Source: CAD feature listing. Evaluate the final solid. Frame: model axes, mm. A direction names the side the tool comes from. Coordinates: 2 decimals unless noted, no trailing zeros. Order: outer loops, then holes, each group sorted by start corner. A loop starts at its lowest first (then second) coordinate and runs counter-clockwise, first axis right, second up.
Item 1: Reachability of faces 4 (the cylindrical face through (-6.4, 0.1, -3.5)), 5 (the cylindrical face through (0, 2, -15)), 6 (the cylindrical face through (6.4, 0.1, -3.5)), 7 (the cylindrical face through (0.1, -6.4, -3.5)) from +Z, -Z, +X, -X, +Y, -Y: full face, straight path, thin tool, end or side. Return the list, or none.
Item 2: Section D-D on z = -8.75. Return the cut outline in (x, y).
Item 3: Section A-A on x = 0. Return the cut outline in (y, z).
Item 4: Ray query, line 1 (Z direction, x = -3.25, y = -7.5); line 2 (Z direction, x = -3, y = -5); line 3 (X direction, y = -2, z = -8.75). Return the intervals inside material, ascending.
Item 5: Contact query for flat-ended pins moving along their axis: P1, Ø0.6, axis at x = -9, y = 9, coming from the -Z side; P2, Ø10, axis at y = -2, z = -12.5, coming from the +X side; P3, Ø4, axis at x = -6.5, z = -10, coming from the +Y side; P4, Ø10, axis at x = -1.5, z = -4.5, coming from the +Y side. Output: stop coordinate, or through.
Item 6: Mould query, pull axis X, two halves, no side actions, for faces 1 (the cylindrical face through (0.1, 6.5, -3.5)), 2 (the flat face through (0, 0, -18)), 3 (the flat face through (-9.25, 0, 1)). Classes: released by +X, released by -X, zero draft, split by the parting line, or undercut.
Item 7: Section C-C on z = -15.25. Return the cut outline in (x, y).
from build123d import *

# Parameters (mm, degrees)
F0_W          = 18.5
F0_H          = 11
F1_DEPTH      = 9.25
F2_DEPTH      = 9.25
F3_R          = 19
F5_DEPTH      = 25.4
F6_DEPTH      = 25.4
F4_R          = 19
F7_DEPTH      = 25.4
F8_DEPTH      = 25.4
F9_R          = 4
F10_DEPTH     = 3.45753
F11_DEPTH     = 7.5
F12_T1_DEPTH  = 11.75
F12_T3_DEPTH  = 17.5
F12_T5_DEPTH  = 17.5
F12_S9_W      = 0.5
F12_S9_H      = 0.5
F12_T10_DEPTH = 0.5
F12_S15_W     = 0.5
F12_S15_H     = 0.5
F12_T16_DEPTH = 0.5
F12_S21_W     = 0.5
F12_S21_H     = 0.5
F12_T22_DEPTH = 0.5
F12_S27_W     = 0.5
F12_S27_H     = 0.5
F12_T28_DEPTH = 0.5
F12_T34_ANGLE = 60.5906744424
F12_T36_ANGLE = 60.5906744424
F12_T38_ANGLE = 60.5906744424
F12_T40_ANGLE = 60.5906744424
F13_R         = 1.9993297739
F14_DEPTH     = 5


# Not quite as in the source:
# - a fillet or chamfer that OpenCascade refuses, or shapes differently, is made with other operations: its cross-section is extruded or revolved along the edge and cut away or added
# - a feature names something its author has since deleted; it is built from what else it names


with BuildPart() as f1:
    # F0 (on Front) → F1 (new body)
    with BuildSketch(Plane.XZ):
        Rectangle(F0_W, F0_H)
    extrude(amount=-F1_DEPTH)

    # F0 (on Front) → F2 (join)
    with BuildSketch(Plane.XZ):
        Rectangle(F0_W, F0_H)
    extrude(amount=F2_DEPTH)

    # F3 (on Front) → F5 (cut)
    with BuildSketch(Plane.XZ):
        with Locations((0, -22.5)):
            Circle(F3_R)
    extrude(amount=-F5_DEPTH, mode=Mode.SUBTRACT)

    # F3 (on Front) → F6 (cut)
    with BuildSketch(Plane.XZ):
        with Locations((0, -22.5)):
            Circle(F3_R)
    extrude(amount=F6_DEPTH, mode=Mode.SUBTRACT)

    # F4 (on Right) → F7 (cut)
    with BuildSketch(Plane.YZ):
        with Locations((0, -22.5)):
            Circle(F4_R)
    extrude(amount=-F7_DEPTH, mode=Mode.SUBTRACT)

    # F4 (on Right) → F8 (cut)
    with BuildSketch(Plane.YZ):
        with Locations((0, -22.5)):
            Circle(F4_R)
    extrude(amount=F8_DEPTH, mode=Mode.SUBTRACT)

    # F9 (on face) → F10 (join)
    with BuildSketch(Plane(origin=(0, 0, -5.5), x_dir=(1, 0, 0), z_dir=(0, 0, -1))):
        Circle(F9_R)
    extrude(amount=-F10_DEPTH)

    # F11 (add): a face of the model
    f11_faces = [f1.faces().sort_by_distance(p)[0] for p in [
        (0, 0, -5.5),
    ]]
    extrude(f11_faces, amount=F11_DEPTH)

    # F12: fillet of radius 0.5 on 13 edges, made by hand

    # F12_s2 → F12_t1 (cut)
    with BuildSketch(Plane.XY.offset(-6.75)):
        with BuildLine():
            ThreePointArc((9.25, -8.75), (9.1035533906, -9.1035533906), (8.75, -9.25))
            Line((8.75, -9.25), (9.25, -9.25))
            Line((9.25, -9.25), (9.25, -8.75))
        make_face()
        with BuildLine():
            ThreePointArc((-9.25, -8.75), (-9.1035533906, -9.1035533906), (-8.75, -9.25))
            Line((-8.75, -9.25), (-9.25, -9.25))
            Line((-9.25, -9.25), (-9.25, -8.75))
        make_face()
        with BuildLine():
            ThreePointArc((9.25, 8.75), (9.1035533906, 9.1035533906), (8.75, 9.25))
            Line((8.75, 9.25), (9.25, 9.25))
            Line((9.25, 9.25), (9.25, 8.75))
        make_face()
        with BuildLine():
            ThreePointArc((-8.75, 9.25), (-9.1035533906, 9.1035533906), (-9.25, 8.75))
            Line((-9.25, 8.75), (-9.25, 9.25))
            Line((-9.25, 9.25), (-8.75, 9.25))
        make_face()
    extrude(amount=F12_T1_DEPTH, mode=Mode.SUBTRACT)

    # F12_s4 → F12_t3 (cut)
    with BuildSketch(Plane.YZ.offset(-8.75)):
        with BuildLine():
            ThreePointArc((-8.75, 5.5), (-9.1035533906, 5.3535533906), (-9.25, 5))
            Line((-9.25, 5), (-9.25, 5.5))
            Line((-9.25, 5.5), (-8.75, 5.5))
        make_face()
        with BuildLine():
            ThreePointArc((9.25, 5), (9.1035533906, 5.3535533906), (8.75, 5.5))
            Line((8.75, 5.5), (9.25, 5.5))
            Line((9.25, 5.5), (9.25, 5))
        make_face()
    extrude(amount=F12_T3_DEPTH, mode=Mode.SUBTRACT)

    # F12_s6 → F12_t5 (cut)
    with BuildSketch(Plane.XZ.offset(-8.75)):
        with BuildLine():
            ThreePointArc((9.25, 5), (9.1035533906, 5.3535533906), (8.75, 5.5))
            Line((8.75, 5.5), (9.25, 5.5))
            Line((9.25, 5.5), (9.25, 5))
        make_face()
        with BuildLine():
            ThreePointArc((-9.25, 5), (-9.1035533906, 5.3535533906), (-8.75, 5.5))
            Line((-8.75, 5.5), (-9.25, 5.5))
            Line((-9.25, 5.5), (-9.25, 5))
        make_face()
    extrude(amount=F12_T5_DEPTH, mode=Mode.SUBTRACT)


with BuildPart() as f12_tool8:
    # F12_s9 → F12_t10 (new body)
    with BuildSketch(Plane.YZ.offset(8.75)):
        with Locations((-9, 5.25)):
            Rectangle(F12_S9_W, F12_S9_H)
    extrude(amount=F12_T10_DEPTH)

    # F12_s11 → F12_t12 (revolve, cut)
    with BuildSketch(Plane(origin=(8.75, -8.75, 5), x_dir=(0, 0.7071067812, -0.7071067812), z_dir=(0, -0.7071067812, -0.7071067812))):
        with BuildLine():
            ThreePointArc((0, -0.5), (0.5, 0), (0, 0.5))
            Line((0, 0.5), (0, -0.5))
        make_face()
    revolve(axis=Axis((8.75, -8.75, 5), (1, 0, 0)), mode=Mode.SUBTRACT)


with BuildPart() as f1_1:
    add(f1.part)

    # F12_t7: cut F12_tool8
    add(f12_tool8.part, mode=Mode.SUBTRACT)


with BuildPart() as f12_tool14:
    # F12_s15 → F12_t16 (new body)
    with BuildSketch(Plane.YZ.offset(-8.75)):
        with Locations((-9, 5.25)):
            Rectangle(F12_S15_W, F12_S15_H)
    extrude(amount=-F12_T16_DEPTH)

    # F12_s17 → F12_t18 (revolve, cut)
    with BuildSketch(Plane(origin=(-8.75, -8.75, 5), x_dir=(0, 0.7071067812, -0.7071067812), z_dir=(0, 0.7071067812, 0.7071067812))):
        with BuildLine():
            ThreePointArc((0, -0.5), (0.5, 0), (0, 0.5))
            Line((0, 0.5), (0, -0.5))
        make_face()
    revolve(axis=Axis((-8.75, -8.75, 5), (-1, 0, 0)), mode=Mode.SUBTRACT)


with BuildPart() as f1_2:
    add(f1_1.part)

    # F12_t13: cut F12_tool14
    add(f12_tool14.part, mode=Mode.SUBTRACT)


with BuildPart() as f12_tool20:
    # F12_s21 → F12_t22 (new body)
    with BuildSketch(Plane.YZ.offset(8.75)):
        with Locations((9, 5.25)):
            Rectangle(F12_S21_W, F12_S21_H)
    extrude(amount=F12_T22_DEPTH)

    # F12_s23 → F12_t24 (revolve, cut)
    with BuildSketch(Plane(origin=(8.75, 8.75, 5), x_dir=(0, -0.7071067812, -0.7071067812), z_dir=(0, -0.7071067812, 0.7071067812))):
        with BuildLine():
            ThreePointArc((0, -0.5), (0.5, 0), (0, 0.5))
            Line((0, 0.5), (0, -0.5))
        make_face()
    revolve(axis=Axis((8.75, 8.75, 5), (1, 0, 0)), mode=Mode.SUBTRACT)


with BuildPart() as f1_3:
    add(f1_2.part)

    # F12_t19: cut F12_tool20
    add(f12_tool20.part, mode=Mode.SUBTRACT)


with BuildPart() as f12_tool26:
    # F12_s27 → F12_t28 (new body)
    with BuildSketch(Plane.XZ.offset(-8.75)):
        with Locations((-9, 5.25)):
            Rectangle(F12_S27_W, F12_S27_H)
    extrude(amount=-F12_T28_DEPTH)

    # F12_s29 → F12_t30 (revolve, cut)
    with BuildSketch(Plane(origin=(-8.75, 8.75, 5), x_dir=(0.7071067812, 0, -0.7071067812), z_dir=(0.7071067812, 0, 0.7071067812))):
        with BuildLine():
            ThreePointArc((0, -0.5), (0.5, 0), (0, 0.5))
            Line((0, 0.5), (0, -0.5))
        make_face()
    revolve(axis=Axis((-8.75, 8.75, 5), (0, 1, 0)), mode=Mode.SUBTRACT)


with BuildPart() as f1_4:
    add(f1_3.part)

    # F12_t25: cut F12_tool26
    add(f12_tool26.part, mode=Mode.SUBTRACT)

    # F12_s31 → F12_t32 (revolve, cut)
    with BuildSketch(Plane.XZ):
        with BuildLine():
            ThreePointArc((4, -12.5), (3.8535533906, -12.8535533906), (3.5, -13))
            Line((3.5, -13), (4, -13))
            Line((4, -13), (4, -12.5))
        make_face()
    revolve(axis=Axis((0, 0, -13), (0, 0, -1)), mode=Mode.SUBTRACT)

    # F12_s33 → F12_t34 (revolve, cut)
    with BuildSketch(Plane(origin=(-9.8002563667, 0, -5.7257375924), x_dir=(0, 1, 0), z_dir=(-0.8634366066, 0, -0.5044573583))):
        with BuildLine():
            ThreePointArc((-8.75, 0.4273236492), (-9.1035533906, 0.2808770398), (-9.25, -0.0726763508))
            Line((-9.25, -0.0726763508), (-9.25, 0.4273236492))
            Line((-9.25, 0.4273236492), (-8.75, 0.4273236492))
        make_face()
    revolve(axis=Axis((0, -9.25, -22.5), (0, 1, 0)), revolution_arc=F12_T34_ANGLE, mode=Mode.SUBTRACT)

    # F12_s35 → F12_t36 (revolve, cut)
    with BuildSketch(Plane(origin=(0, 9.8002563667, -5.7257375924), x_dir=(1, 0, 0), z_dir=(0, 0.8634366066, -0.5044573583))):
        with BuildLine():
            ThreePointArc((-9.25, -0.0726763508), (-9.1035533906, 0.2808770398), (-8.75, 0.4273236492))
            Line((-8.75, 0.4273236492), (-9.25, 0.4273236492))
            Line((-9.25, 0.4273236492), (-9.25, -0.0726763508))
        make_face()
    revolve(axis=Axis((-9.25, 0, -22.5), (1, 0, 0)), revolution_arc=F12_T36_ANGLE, mode=Mode.SUBTRACT)

    # F12_s37 → F12_t38 (revolve, cut)
    with BuildSketch(Plane(origin=(0, -9.8002563667, -5.7257375924), x_dir=(1, 0, 0), z_dir=(0, -0.8634366066, -0.5044573583))):
        with BuildLine():
            ThreePointArc((9.25, 0.0726763508), (9.1035533906, -0.2808770398), (8.75, -0.4273236492))
            Line((8.75, -0.4273236492), (9.25, -0.4273236492))
            Line((9.25, -0.4273236492), (9.25, 0.0726763508))
        make_face()
    revolve(axis=Axis((9.25, 0, -22.5), (-1, 0, 0)), revolution_arc=F12_T38_ANGLE, mode=Mode.SUBTRACT)

    # F12_s39 → F12_t40 (revolve, cut)
    with BuildSketch(Plane(origin=(9.8002563667, 0, -5.7257375924), x_dir=(0, 1, 0), z_dir=(0.8634366066, 0, -0.5044573583))):
        with BuildLine():
            ThreePointArc((9.25, 0.0726763508), (9.1035533906, -0.2808770398), (8.75, -0.4273236492))
            Line((8.75, -0.4273236492), (9.25, -0.4273236492))
            Line((9.25, -0.4273236492), (9.25, 0.0726763508))
        make_face()
    revolve(axis=Axis((0, 9.25, -22.5), (0, -1, 0)), revolution_arc=F12_T40_ANGLE, mode=Mode.SUBTRACT)

    # F13 (on face) → F14 (join)
    with BuildSketch(Plane(origin=(0, 0, -13), x_dir=(1, 0, 0), z_dir=(0, 0, -1))):
        Circle(F13_R)
    extrude(amount=F14_DEPTH)


solid = f1_4.part
Answer list:
1. face 4: -Z, -X
1. face 5: -Z
1. face 6: -Z, +X
1. face 7: -Z, -Y
2. outline: circle Ø8 at (0, 0)
3. outline: (-9.25, -3) arc R0.5 ccw to (-8.75, -3.5) - (-4, -3.5) - (-4, -12.5) arc R0.5 ccw to (-3.5, -13) - (-2, -13) - (-2, -18) - (2, -18) - (2, -13) - (3.5, -13) arc R0.5 ccw to (4, -12.5) - (4, -3.5) - (8.75, -3.5) arc R0.5 ccw to (9.25, -3) - (9.25, 5) arc R0.5 ccw to (8.75, 5.5) - (-8.75, 5.5) arc R0.5 ccw to (-9.25, 5) - close
4. line 1: z = -3.78 to 5.5
4. line 2: z = -3.74 to 5.5
4. line 3: x = -3.46 to 3.46
5. P1: stops at z = -5.5
5. P2: stops at x = 4
5. P3: passes through
5. P4: stops at y = 9.25
6. face 1: undercut
6. face 2: zero draft
6. face 3: released by -X
7. outline: circle Ø4 at (0, 0)
